from build123d import *

# Parameters (mm, degrees)
SKETCH1_R           = 1.5
BOSS_EXTRUDE1_DEPTH = 3


with BuildPart() as part:
    # Sketch1 → Boss-Extrude1 (new body)
    with BuildSketch(Plane.XY):
        with BuildLine():
            ThreePointArc((16.667258487, 3.092264578), (2.252499278, 7.520108125), (-12.291231068, 3.536267122))
            ThreePointArc((-12.291231068, 3.536267122), (-13.280504589, -0.589425292), (-9.154812174, -1.578698813))
            ThreePointArc((-9.154812174, -1.578698813), (2.160515814, 1.520813246), (13.375501545, -1.924142128))
            ThreePointArc((13.375501545, -1.924142128), (17.529583369, -1.061817246), (16.667258487, 3.092264578))
        make_face()
        with Locations((-10.723021621, 0.978784155)):
            Circle(SKETCH1_R, mode=Mode.SUBTRACT)
        with Locations((15.021380016, 0.584061225)):
            Circle(SKETCH1_R, mode=Mode.SUBTRACT)
    extrude(amount=BOSS_EXTRUDE1_DEPTH)


solid = part.part
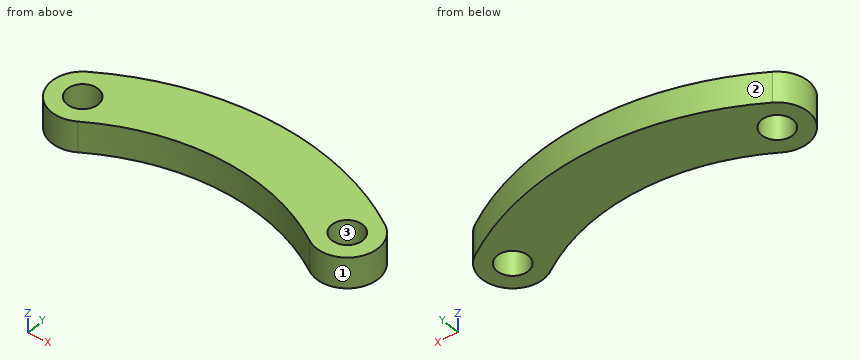
Input: part model. Units: mm. Frame: model coordinates. Face numbers are marked on the shaded views. Coordinates: 2 decimals unless noted, no trailing zeros. Loops run counter-clockwise (first coordinate to the right, second up) from the corner with the lowest first, then second, coordinate; pieces in that order, holes last. Notation, with made-up numbers: (-19.5, 2.25) - (5.5, 2.25) arc R22 ccw to (5.5, 25.25) - close; hole circle Ø6 at (15, 65). An arc over 180 degrees is marked (long way). Answer in a Markdown table with one row per item. Add a question column.
Item 1: Section query C-C on z = 2.25. Return the cut outline in (x, y).
Item 2: Line query: line 1 along X through (y, z) = (0, 1.4); line 2 along X through (y, z) = (1.75, 2.2); line 3 along X through (y, z) = (2.25, 2.3). Output: solid intervals per line, ascending. Write a range as [from, to].
Item 3: Section query A-A on x = 14. Return the cut outline in (y, z).
Item 4: Section query D-D on x = 9. Return the cut outline in (y, z).
Item 5: Section query B-B on y = -0.25. Return the cut outline in (x, z), then the cut area to 3 significant figures.
Item 6: Contact query for flat-ended pins moving along their axis: P1, Ø2.5, axis at x = 15.02, y = 0.58, coming from the +Z side; P2, Ø1.5, axis at x = 12.5, z = 2.5, coming from the +Y side. Output: stop coordinate, or through.
Item 7: Mould query, pull axis Y, two halves, no side actions, for the marked faces 1, 2 and 3. Classes: released by +Y, released by -Y, zero draft, split by the parting line, or undercut.
Recorded:
| question | item | result |
|---|---|---|
| 1 | outline | (-12.29, 3.54) arc R3 ccw to (-9.15, -1.58) arc R21.03 cw to (13.38, -1.92) arc R3 ccw to (16.67, 3.09) arc R27.03 ccw to start; hole circle Ø3 at (-10.72, 0.98); hole circle Ø3 at (15.02, 0.58) |
| 2 | line 1 | [-13.56, -11.86], [-9.59, -6.02], [9.7, 13.64], [16.4, 17.96] |
| 2 | line 2 | [-13.62, -12.01], [-9.44, 14.08], [15.97, 17.79] |
| 2 | line 3 | [-13.44, -11.52], [-9.93, 17.52] |
| 3 | outline | (-2.24, 0) - (-0.51, 0) - (-0.51, 3) - (-2.24, 3) - close; (1.68, 0) - (4.63, 0) - (4.63, 3) - (1.68, 3) - close |
| 4 | outline | (0.27, 0) - (6.56, 0) - (6.56, 3) - (0.27, 3) - close |
| 5 | outline | (-13.46, 0) - (-11.58, 0) - (-11.58, 3) - (-13.46, 3) - close; (-9.86, 0) - (-6.61, 0) - (-6.61, 3) - (-9.86, 3) - close; (10.29, 0) - (13.77, 0) - (13.77, 3) - (10.29, 3) - close; (16.27, 0) - (17.9, 0) - (17.9, 3) - (16.27, 3) - close |
| 5 | area | 30.7 mm^2 |
| 6 | P1 | through |
| 6 | P2 | y = 5.64 |
| 7 | face 1 | split by the parting line |
| 7 | face 2 | released by +Y |
| 7 | face 3 | undercut |
